Can you work these out from the model? Positions are in its coordinate system, mm. Face numbers are marked on the shaded views. A direction names the side the tool comes from. Coordinates: 2 decimals unless noted, no trailing zeros. Order: outer loops, then holes, each group sorted by start corner. A loop starts at its lowest first (then second) coordinate and runs counter-clockwise, first axis right, second up. Notation, with made-up numbers: M 42.25,-29.5 L 80.25,-29.5 A22 ccw 80.25,-20.5 Z; hole C 61,18.25 d3. An arc over 180 degrees is marked long. Answer as a JSON object with one key per item and string values.
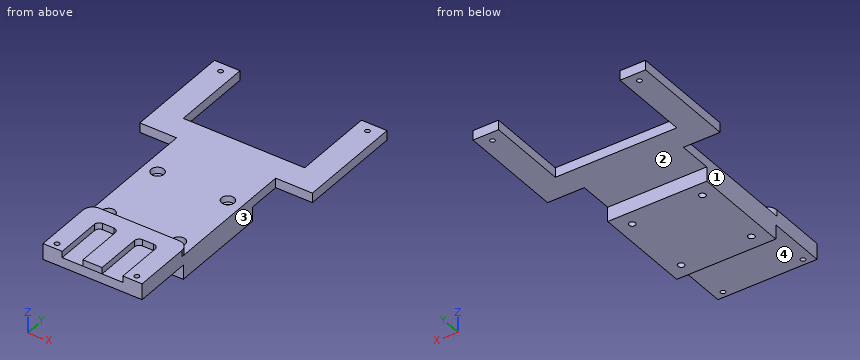
from build123d import *

# Parameters (mm, degrees)
SKETCH_R        = 1.5
PAD_DEPTH       = 6
PAD001_DEPTH    = 4
SKETCH002_R     = 1.5
POCKET_DEPTH    = 10
SKETCH003_W     = 62
SKETCH003_H     = 62
PAD002_DEPTH    = 9
SKETCH004_R     = 2
POCKET001_DEPTH = 15
SKETCH005_R     = 4
POCKET002_DEPTH = 4


with BuildPart() as part:
    # Sketch → Pad (new body)
    with BuildSketch(Plane.XY):
        Polygon((-38, 29), (38, 29), (38, 80), (54, 80), (54, 13), (31, 13), (31, -107), (-31, -107), (-31, 13), (-54, 13), (-54, 80), (-38, 80), align=None)
        with Locations((46, 74)):
            Circle(SKETCH_R, mode=Mode.SUBTRACT)
        with Locations((-46, 74)):
            Circle(SKETCH_R, mode=Mode.SUBTRACT)
    extrude(amount=PAD_DEPTH)

    # Sketch001 (on Face16 of Pad) → Pad001 (join)
    with BuildSketch(Plane.XY.offset(6)):
        with BuildLine():
            Line((31, -71), (31, -107))
            Line((19, -107), (31, -107))
            Line((19, -78.000015), (19, -107))
            ThreePointArc((19, -78.000015), (18.12132, -75.878696), (16.000001, -75.000016))
            Line((8.999999, -75.000016), (16.000001, -75.000016))
            ThreePointArc((8.999999, -75.000016), (6.878678, -75.878697), (6, -78.000019))
            Line((6, -107.000009), (6, -78.000019))
            Line((-6, -107.000009), (6, -107.000009))
            Line((-6, -78.000019), (-6, -107.000009))
            ThreePointArc((-6, -78.000019), (-6.878676, -75.878693), (-8.999999, -75.000009))
            Line((-16.000001, -75.000009), (-8.999999, -75.000009))
            ThreePointArc((-16.000001, -75.000009), (-18.12132, -75.878689), (-19, -78.000009))
            Line((-19, -107), (-19, -78.000009))
            Line((-31, -107), (-19, -107))
            Line((-31, -107), (-31, -71))
            ThreePointArc((-25, -65), (-29.242641, -66.757359), (-31, -71))
            Line((-25, -65), (25, -65))
            ThreePointArc((31, -71), (29.242641, -66.757359), (25, -65))
        make_face()
    extrude(amount=PAD001_DEPTH)

    # Sketch002 (on Face27 of Pad001) → Pocket (cut)
    with BuildSketch(Plane.XY.offset(10)):
        with Locations((-25, -103)):
            Circle(SKETCH002_R)
        with Locations((25, -103)):
            Circle(SKETCH002_R)
    extrude(amount=-POCKET_DEPTH, mode=Mode.SUBTRACT)

    # Sketch003 (on Face4 of Pocket) → Pad002 (join)
    with BuildSketch(Plane(origin=(0, 0, 0), x_dir=(1, 0, 0), z_dir=(0, 0, -1))):
        with Locations((0, 39)):
            Rectangle(SKETCH003_W, SKETCH003_H)
    extrude(amount=PAD002_DEPTH)

    # Sketch004 (on Face25 of Pad002) → Pocket001 (cut)
    with BuildSketch(Plane(origin=(0, 0, -9), x_dir=(1, 0, 0), z_dir=(0, 0, -1))):
        with Locations((-22, 61)):
            Circle(SKETCH004_R)
        with Locations((22, 61)):
            Circle(SKETCH004_R)
        with Locations((22, 17)):
            Circle(SKETCH004_R)
        with Locations((-22, 17)):
            Circle(SKETCH004_R)
    extrude(amount=-POCKET001_DEPTH, mode=Mode.SUBTRACT)

    # Sketch005 (on Face5 of Pocket001) → Pocket002 (cut)
    with BuildSketch(Plane.XY.offset(6)):
        with Locations((-22, -61)):
            Circle(SKETCH005_R)
        with Locations((22, -61)):
            Circle(SKETCH005_R)
        with Locations((22, -17)):
            Circle(SKETCH005_R)
        with Locations((-22, -17)):
            Circle(SKETCH005_R)
    extrude(amount=-POCKET002_DEPTH, mode=Mode.SUBTRACT)


solid = part.part
Item 1: I want a section at A-A, the plane y = -61. Write out the boundary of the cut face in (x, z), plus the area to 3 significant figures.
Answers follow:
{"outline": "M -31,-9 L -24,-9 L -24,2 L -26,2 L -26,6 L -31,6 Z; M -20,-9 L 20,-9 L 20,2 L 18,2 L 18,6 L -18,6 L -18,2 L -20,2 Z; M 24,-9 L 31,-9 L 31,6 L 26,6 L 26,2 L 24,2 Z", "area": "778 mm^2"}
Item 2: Which directions (+Z, -Z, +X, -X, +Y, -Y) give clear straight access to the entire face, cutting with the end or side of a thin tool? Please do the marked faces 1, 2, 3 and 4.
Answers follow:
{"face 1": "+Z, -Z, -X, -Y", "face 2": "-Z, +X, -X, +Y", "face 3": "+Z, -Z, +X, -Y", "face 4": "-Z, +X, -X, -Y"}
Item 3: Please list where these lines run through material, in increasing order: line 1 (Y direction, x = 22, z = -3.25); line 2 (X direction, y = -103, z = 7.25); line 3 (X direction, y = -61, z = -6.5).
Answers follow:
{"line 1": "y = -70 to -63, -59 to -19, -15 to -8", "line 2": "x = -31 to -26.5, -23.5 to -19, -6 to 6, 19 to 23.5, 26.5 to 31", "line 3": "x = -31 to -24, -20 to 20, 24 to 31"}
Item 4: I want a section at C-C, the plane x = 29. Write out the boundary of the cut face in (y, z).
Answers follow:
{"outline": "M -107,0 L -70,0 L -70,-9 L -8,-9 L -8,0 L 29,0 L 29,6 L -66.53,6 L -66.53,10 L -107,10 Z"}
Item 5: I want a section at D-D, the plane y = -30.5. Write out the boundary of the cut face in (x, z).
Answers follow:
{"outline": "M -31,-9 L 31,-9 L 31,6 L -31,6 Z"}
Item 6: I'm going to push flat-ended pins straight in: pin 1 (5 mm diameter, centred on x = 47.5, z = 3.5, fed in from -Y); pin 2 (6.5 mm diameter, centred on x = -21, y = -18, fed in from +Z); pin 3 (3 mm diameter, centred on x = -14.5, z = 3.5, fed in from +Y). Where does each tip first touch, or does it pass through?
Answers follow:
{"pin 1": "stops at y = 13", "pin 2": "stops at z = 6", "pin 3": "stops at y = 29"}
Item 7: I want a section at B-B, the plane y = 35. Write out the boundary of the cut face in (x, z).
Answers follow:
{"outline": "M -54,0 L -38,0 L -38,6 L -54,6 Z; M 38,0 L 54,0 L 54,6 L 38,6 Z"}
